Input: part model. Units: mm. Frame: model coordinates. Round coordinates to 2 decimals unless told otherwise and drop trailing zeros. Loops run counter-clockwise (first coordinate to the right, second up) from the corner with the lowest first, then second, coordinate; pieces in that order, holes last. Notation, with made-up numbers: (81, 75) -> (140, 75) arc R3 ccw to (140, 79) -> close; hole circle Ø6 at (-34.5, 10.25). An arc over 180 degrees is marked (long way). Answer in a Markdown table with one row per item. Add a question column.
Q1. Ray query, L1, parallel to X at y = 23, z = 1.85; L2, parallel to X at y = 13.5, z = 1.25. Return the intervals inside material, ascending. Write a range as from..to.
Q2. Section B-B, the plane z = 1.85. Output: boundary loops of the cut face in (x, y).
Q3. Mould query, pull axis Y, two halves, no side actions, for faces 1 (the face through (187.955, 27.305, 1.602)), 2 (the face through (41, 27, 3.16)). Classes: pulls with the +Y half, pulls with the -Y half, needs draft (parallel to the pull), parting line crosses it, or undercut.
Q4. Section A-A, the plane y = 14. Output: boundary loops of the cut face in (x, z).
Q5. Section C-C, the plane y = 31. Output: boundary loops of the cut face in (x, z), and give its area (3 significant figures).
```python
from build123d import *

# Parameters (mm, degrees)
SKETCH2_W           = 77.34
SKETCH2_H           = 87.37
BOSS_EXTRUDE1_DEPTH = 3.16
SKETCH_3_W          = 3.16
SKETCH_3_H          = 87.37
EXTRUDE_3_DEPTH     = 80
SKETCH_4_W          = 3.16
SKETCH_4_H          = 87.37
EXTRUDE_4_DEPTH     = 60
SKETCH_5_W          = 3.16
SKETCH_5_H          = 87.37
EXTRUDE_5_DEPTH     = 113
SKETCH_6_W          = 3.16
SKETCH_6_H          = 87.37
CUT_EXTRUDE_1_DEPTH = 17.86
SKETCH_8_R          = 12.75
CUT_EXTRUDE_2_DEPTH = 10


with BuildPart() as part:
    # Sketch2 → Boss-Extrude1 (new body)
    with BuildSketch(Plane.XY):
        with Locations((-14.294928595, 27.706753385)):
            Rectangle(SKETCH2_W, SKETCH2_H)
    extrude(amount=BOSS_EXTRUDE1_DEPTH)

    # 草图3 → 凸台-拉伸3 (add)
    with BuildSketch(Plane(origin=(24.375071405, 0, 0), x_dir=(0, 0, -1), z_dir=(1, 0, 0))):
        with Locations((-1.58, 27.706753385)):
            Rectangle(SKETCH_3_W, SKETCH_3_H)
    extrude(amount=EXTRUDE_3_DEPTH)

    # 草图4 → 凸台-拉伸4 (add)
    with BuildSketch(Plane.ZY.offset(52.964928595)):
        with Locations((1.58, 27.706753385)):
            Rectangle(SKETCH_4_W, SKETCH_4_H)
    extrude(amount=EXTRUDE_4_DEPTH)

    # 草图5 → 凸台-拉伸5 (add)
    with BuildSketch(Plane(origin=(104.375071405, 0, 0), x_dir=(0, 0, -1), z_dir=(1, 0, 0))):
        with Locations((-1.58, 27.706753385)):
            Rectangle(SKETCH_5_W, SKETCH_5_H)
    extrude(amount=EXTRUDE_5_DEPTH)

    # 草图6 → 切除-拉伸1 (cut)
    with BuildSketch(Plane(origin=(217.375071405, 0, 0), x_dir=(0, 0, -1), z_dir=(1, 0, 0))):
        with Locations((-1.58, 27.706753385)):
            Rectangle(SKETCH_6_W, SKETCH_6_H)
    extrude(amount=-CUT_EXTRUDE_1_DEPTH, mode=Mode.SUBTRACT)

    # 草图8 → 切除-拉伸2 (cut)
    with BuildSketch(Plane.XY.offset(3.16)):
        with Locations((175.79355983, 23.47529756)):
            Circle(SKETCH_8_R)
    extrude(amount=-CUT_EXTRUDE_2_DEPTH, mode=Mode.SUBTRACT)


solid = part.part
```
Answer block:
| question | item | result |
|---|---|---|
| 1 | L1 | -112.96..163.05, 188.53..199.52 |
| 1 | L2 | -112.96..167.85, 183.73..199.52 |
| 2 | outline | (-112.96, -15.98) -> (199.52, -15.98) -> (199.52, 71.39) -> (-112.96, 71.39) -> close; hole circle Ø25.5 at (175.79, 23.48) |
| 3 | face 1 | undercut |
| 3 | face 2 | needs draft |
| 4 | outline | (-112.96, 0) -> (167.26, 0) -> (167.26, 3.16) -> (-112.96, 3.16) -> close; (184.32, 0) -> (199.52, 0) -> (199.52, 3.16) -> (184.32, 3.16) -> close |
| 5 | outline | (-112.96, 0) -> (165.5, 0) -> (165.5, 3.16) -> (-112.96, 3.16) -> close; (186.09, 0) -> (199.52, 0) -> (199.52, 3.16) -> (186.09, 3.16) -> close |
| 5 | area | 922 mm^2 |
